from build123d import *

# Parameters (mm, degrees)
CUT_EXTRUDE1_DEPTH = 1.905
CUT_EXTRUDE2_REACH = 12.17
SKETCH3_R          = 1.27
SKETCH4_R          = 2.3495
CUT_EXTRUDE3_DEPTH = 6.35
FILLET1_R          = 3.175


with BuildPart() as part:
    # Sketch1 → Revolve1 (revolve)
    with BuildSketch(Plane.XY, mode=Mode.PRIVATE) as revolve1_sk:
        Polygon((0, 0), (-3.175, 0), (-3.175, 6.35), (-4.7625, 6.35), (-4.7625, 9.525), (0, 9.525), align=None)
    revolve(revolve1_sk.sketch.rotate(Axis((0, 9.525, 0), (0, -1, 0)), 270), axis=Axis((0, 9.525, 0), (0, -1, 0)))

    # Sketch2 → Cut-Extrude1 (cut)
    with BuildSketch(Plane(origin=(0, 9.525, 0), x_dir=(1, 0, 0), z_dir=(0, 1, 0))):
        Polygon((-1.374815329, -2.38125), (1.374815329, -2.38125), (2.749630657, 0), (1.374815329, 2.38125), (-1.374815329, 2.38125), (-2.749630657, 0), align=None)
    extrude(amount=-CUT_EXTRUDE1_DEPTH, mode=Mode.SUBTRACT)

    # Sketch3 → Cut-Extrude2 (cut, up to next)
    with BuildSketch(Plane(origin=(0, 7.62, 0), x_dir=(1, 0, 0), z_dir=(0, 1, 0)), mode=Mode.PRIVATE) as cut_extrude2_sk1:
        with Locations(Location((0, 0, 0), (0, 0, 270))):
            Circle(SKETCH3_R)
    cut_extrude2_tool1 = extrude(cut_extrude2_sk1.sketch, amount=-CUT_EXTRUDE2_REACH, mode=Mode.PRIVATE) & part.part
    add(cut_extrude2_tool1.solids().sort_by_distance((0, 7.62, 0))[0], mode=Mode.SUBTRACT)

    # Sketch4 → Cut-Extrude3 (cut)
    with BuildSketch(Plane.XZ):
        with Locations(Location((0, 0, 0), (0, 0, 270))):
            Circle(SKETCH4_R)
    extrude(amount=-CUT_EXTRUDE3_DEPTH, mode=Mode.SUBTRACT)

    # Fillet1
    # the kernel refuses this fillet: 3.175 mm, written as the material it takes off along each edge
    with BuildSketch(Plane(origin=(0, 9.525, 0), x_dir=(0, 0, 1), z_dir=(1, 0, 0))) as fillet1_piece_1:
        with BuildLine():
            CenterArc((4.7625 - FILLET1_R, FILLET1_R), FILLET1_R, 270, 90)
            Line((4.7625 - FILLET1_R, 0), (4.7625, 0))
            Line((4.7625, 0), (4.7625, FILLET1_R))
        make_face()
    revolve(axis=Axis((0, 9.525, 0), (0, -1, 0)), mode=Mode.SUBTRACT)


solid = part.part
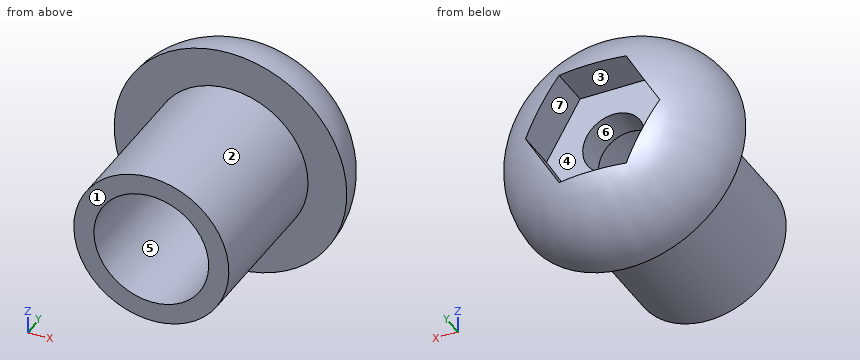
Geometry check sheet. Reference: the model listing, model coordinates, mm. Face numbers are marked on the shaded views. A direction names the side the tool comes from. Give positions to 0.01 mm unless a question says otherwise; leave off trailing zeros. Answer as a JSON object with one key per item and string values.
(1) Depth check by flat-ended pin: pin 1 Ø2 at (x, z) = (-0.5, -0.5) entering from +Y; pin 2 Ø1 at (x, y) = (2, 1.5) entering from +Z; pin 3 Ø3 at (x, z) = (0, 2) entering from -Y; pin 4 Ø4 at (x, z) = (0, 0) entering from -Y. Enter the tip coordinate at first touch or a pass-through.
Report:
{"pin 1": "y = 7.62", "pin 2": "z = 2.8", "pin 3": "y = 0", "pin 4": "y = 6.35"}
(2) Material ranges on line 1 (X direction, y = 3.25, z = 0) (1 decimal); line 2 (X direction, y = 6.6, z = 0); line 3 (Z direction, x = -0.5, y = 3), recorded low to high.
Report:
{"line 1": "-3.2 to -2.3, 2.3 to 3.2", "line 2": "-4.75 to -1.27, 1.27 to 4.75", "line 3": "-3.14 to -2.3, 2.3 to 3.14"}
(3) Tool access check on the marked faces 5, 6 and 7. Record the directions out of +Z, -Z, +X, -X, +Y, -Y that give a thin tool (end or side, any length) a straight path to the whole face; none if there is none.
Report:
{"face 5": "-Y", "face 6": "+Y, -Y", "face 7": "+Y"}
(4) Draft check along X on the marked faces 1, 2, 3 and 4. Enter one of: released by +X, released by -X, zero draft, split by the parting line, or undercut.
Report:
{"face 1": "zero draft", "face 2": "split by the parting line", "face 3": "undercut", "face 4": "undercut"}
